Print and shaded views of the part. All mm, measured from the part's lowest x, y and z. A direction names the side the tool comes from. Round coordinates to 2 decimals unless told otherwise and drop trailing zeros. Order: outer loops, then holes, each group sorted by start corner. A loop starts at its lowest first (then second) coordinate and runs counter-clockwise, first axis right, second up. Notation, with made-up numbers: (59, 68) - (94, 68) arc R30 cw to (94, 99) - close; hole circle Ø7 at (77, -19.5). An arc over 180 degrees is marked (long way). Return JSON: item names as keys, results as strings. Group by question number.
Item 1: Saw through at C-C on y = 7. List the corners of the cut face in (x, z).
Item 2: Saw through at A-A on x = 12. List the corners of the cut face in (y, z), and give its area (3 significant figures).
Item 3: Saw through at B-B on z = 12. List the corners of the cut face in (x, y).
Item 4: Drop flat-ended pins along their axis: pin 1 (4 mm diameter, centred on y = 10.5, z = 6, fed in from +X); pin 2 (3 mm diameter, centred on x = 18, y = 3, fed in from -Z); pin 3 (3 mm diameter, centred on x = 6.5, y = 8, fed in from +Z); pin 4 (8 mm diameter, centred on x = 9.5, z = 5, fed in from -Y). Give the stop position or say it passes through.
Item 5: Probe probe 1 along Y at (x, z) = (12, 9.75); probe 2 along Y at (x, z) = (12.5, 21); probe 3 along X at (y, z) = (7, 11). List the from-to ranges inside material, lowest first.
Item 6: Saw through at D-D on x = 17.25. List the corners of the cut face in (y, z), and give its area (3 significant figures).
Item 7: Tool access for the marked faces 1 and 2: list every direction of +Z, -Z, +X, -X, +Y, -Y with a clear straight run to the whole face (end or side of a thin tool).
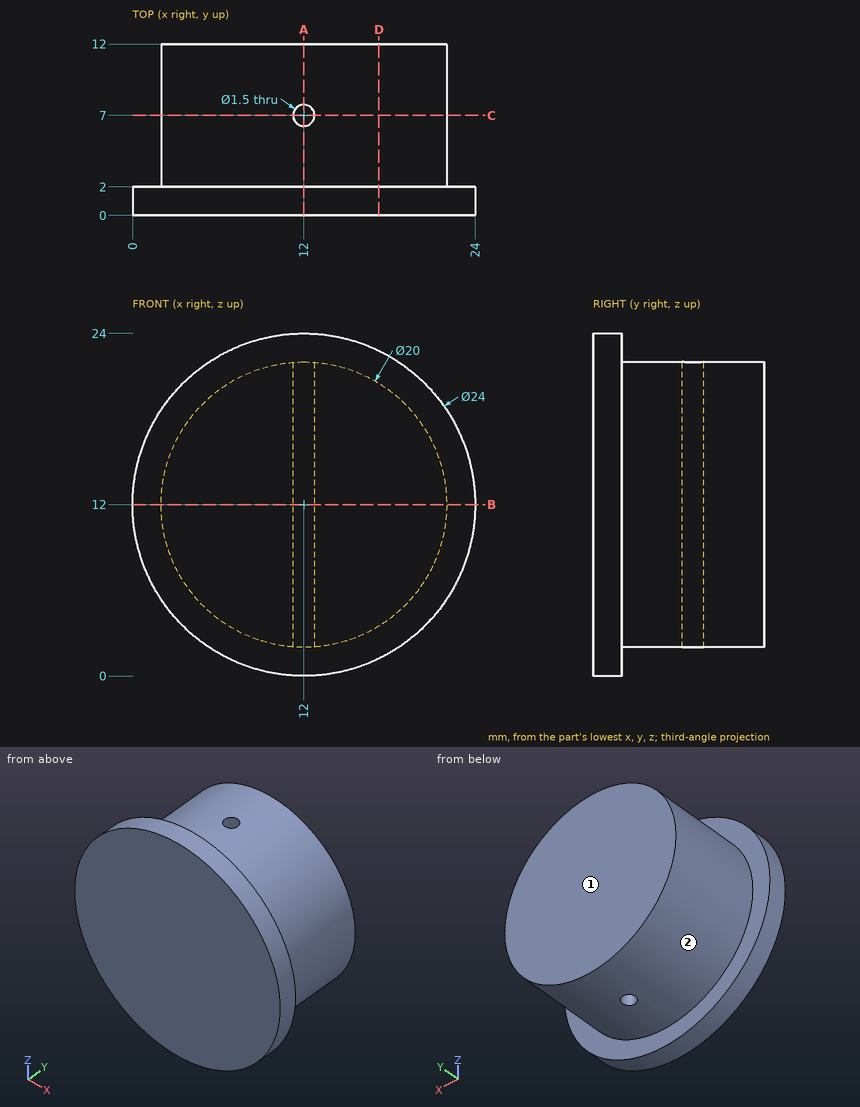
Filled in:
{
 "1": {"outline": "(11.25, 2.03) - (11.25, 21.97) arc R10 ccw to start; (12.75, 2.03) arc R10 ccw to (12.75, 21.97) - close"},
 "2": {"outline": "(0, 0) - (2, 0) - (2, 2) - (6.25, 2) - (6.25, 22) - (2, 22) - (2, 24) - (0, 24) - close; (7.75, 2) - (12, 2) - (12, 22) - (7.75, 22) - close", "area": "218 mm^2"},
 "3": {"outline": "(0, 0) - (24, 0) - (24, 2) - (22, 2) - (22, 12) - (2, 12) - (2, 2) - (0, 2) - close; hole circle Ø1.5 at (12, 7)"},
 "4": {"pin 1": "stops at x = 21.17", "pin 2": "stops at z = 1.04", "pin 3": "stops at z = 21.17", "pin 4": "stops at y = 0"},
 "5": {"probe 1": "y = 0 to 6.25, 7.75 to 12", "probe 2": "y = 0 to 6.44, 7.56 to 12", "probe 3": "x = 2.05 to 11.25, 12.75 to 21.95"},
 "6": {"outline": "(0, 1.21) - (2, 1.21) - (2, 3.49) - (12, 3.49) - (12, 20.51) - (2, 20.51) - (2, 22.79) - (0, 22.79) - close", "area": "213 mm^2"},
 "7": {"face 1": "+Z, -Z, +X, -X, +Y", "face 2": "+Y"}
}
